Verification items for this drawing (mm, ordinates from the low corner). A direction names the side the tool comes from. Coordinates: 2 decimals unless noted, no trailing zeros. Order: outer loops, then holes, each group sorted by start corner. A loop starts at its lowest first (then second) coordinate and runs counter-clockwise, first axis right, second up. Notation, with made-up numbers: M 85,-1.5 L 126,-1.5 A22 ccw 126,22.5 Z; hole C 64.25,79.5 d6. An arc over 180 degrees is marked long. One line per item, written item: value. Start each with the question number.
1) Thickness scan on L1, parallel to X at y = 1.75, z = 1.65; L2, parallel to X at y = 17.5, z = 1.35. Record the ranges inside material, lowest first. Write a range as from..to.
2) Draft check along Y on the marked faces 4, 5 and 6. Enter one of: pulls with the +Y half, pulls with the -Y half, needs draft (parallel to the pull), parting line crosses it, or undercut.
3) Sectioned sample at C-C, the plane z = 2.9. Enter the section's corners in (x, y), then the cut area to 3 significant figures.
4) Access from +Z, -Z, +X, -X, +Y, -Y to the whole of each face (thin tool, end or side, straight path). Record for the marked faces 1, 2 and 3.
5) Go/stop test with flat-tipped pins: P1, Ø1.8, axis at x = 13.5, z = 1, coming from the +Y side; P2, Ø1, axis at x = 10.5, z = 3, coming from the -Y side; P3, Ø1.8, axis at y = 11, z = 1.5, coming from the -X side. Record where each tip stops, or that it passes through.
6) Sectioned sample at A-A, the plane x = 23.75. Enter the section's corners in (y, z).
7) Sectioned sample at D-D, the plane y = 15.25. Enter the section's corners in (x, z), then the cut area to 3 significant figures.
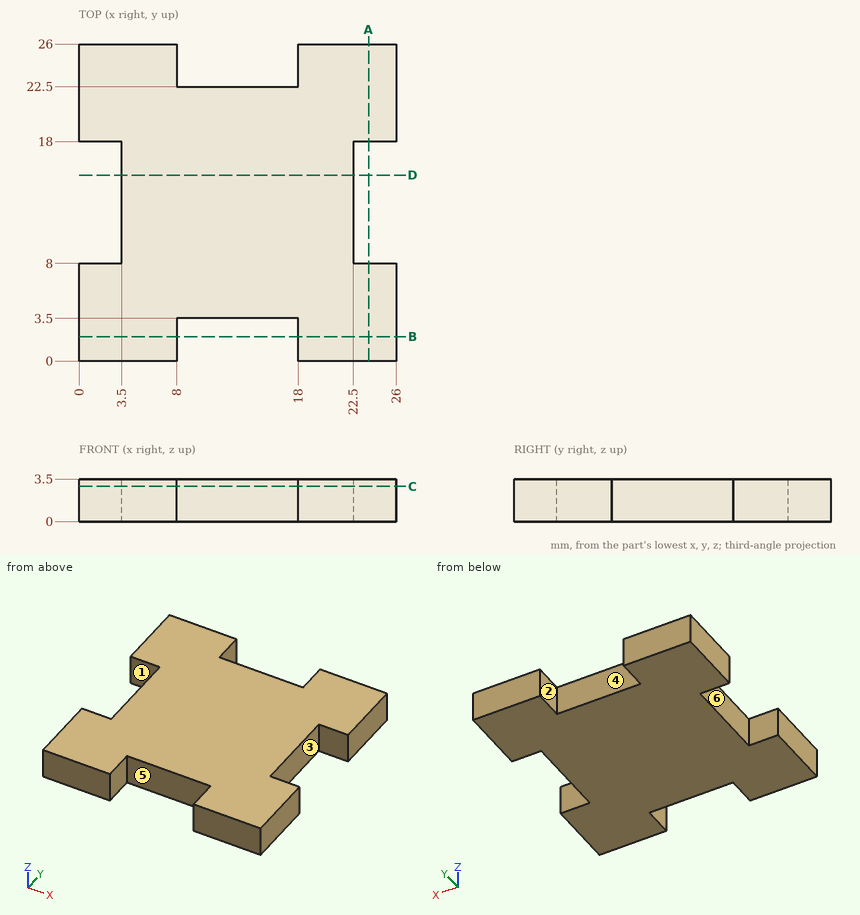
Final values:
1. L1: x = 0..8, 18..26
1. L2: x = 3.5..22.5
2. face 4: pulls with the +Y half
2. face 5: pulls with the -Y half
2. face 6: undercut
3. outline: M 0,0 L 8,0 L 8,3.5 L 18,3.5 L 18,0 L 26,0 L 26,8 L 22.5,8 L 22.5,18 L 26,18 L 26,26 L 18,26 L 18,22.5 L 8,22.5 L 8,26 L 0,26 L 0,18 L 3.5,18 L 3.5,8 L 0,8 Z
3. area: 536 mm^2
4. face 1: +Z, -Z, -X
4. face 2: +Z, -Z, +Y
4. face 3: +Z, -Z, +X
5. P1: stops at y = 22.5
5. P2: stops at y = 3.5
5. P3: stops at x = 3.5
6. outline: M 0,0 L 8,0 L 8,3.5 L 0,3.5 Z; M 18,0 L 26,0 L 26,3.5 L 18,3.5 Z
7. outline: M 3.5,0 L 22.5,0 L 22.5,3.5 L 3.5,3.5 Z
7. area: 66.5 mm^2
